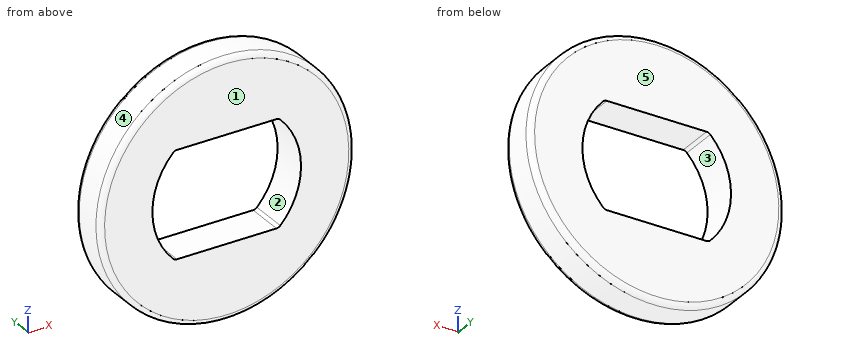
from build123d import *

# Parameters (mm, degrees)
SKETCH_1_R          = 12
EXTRUDE_1_DEPTH     = 3.5
CUT_EXTRUDE_1_DEPTH = 18.327723451
FILLET_1_R          = 0.5


with BuildPart() as part:
    # 草图1 → 凸台-拉伸1 (new body)
    with BuildSketch(Plane(origin=(0, 0, 0), x_dir=(1, 0, 0), z_dir=(0, 1, 0))):
        with Locations(Location((0, 0, 0), (0, 0, 270))):
            Circle(SKETCH_1_R)
    extrude(amount=EXTRUDE_1_DEPTH)

    # 草图2 → 切除-拉伸1 (cut, through all)
    with BuildSketch(Plane.XZ):
        with BuildLine():
            Line((4.898979486, -5), (-4.898979486, -5))
            ThreePointArc((-4.898979486, -5), (-7, 0), (-4.898979486, 5))
            Line((-4.898979486, 5), (4.898979486, 5))
            ThreePointArc((4.898979486, 5), (7, 0), (4.898979486, -5))
        make_face()
    extrude(amount=-CUT_EXTRUDE_1_DEPTH, mode=Mode.SUBTRACT)

    # 圆角1
    fillet_1_edges = [part.edges().sort_by_distance(p)[0] for p in [
        (4.898979486, 1.75, -5),
        (-4.898979486, 1.75, -5),
        (-4.898979486, 1.75, 5),
        (0, 0, -12),
        (0, 3.5, -12),
        (4.898979486, 1.75, 5),
    ]]
    fillet(fillet_1_edges, radius=FILLET_1_R)


solid = part.part
Can you work these out from the model? Positions are in its coordinate system, mm. Face numbers are marked on the shaded views. A direction names the side the tool comes from. Coordinates: 2 decimals unless noted, no trailing zeros. Write each loop counter-clockwise with the first axis right and the second up, starting at its lowest first coordinate (ties: lowest second). Pieces come first, ordered by that corner, then holes. Notation, with made-up numbers: (49.25, 45.5) -> (74.25, 45.5) arc R24 cw to (74.25, 77.5) -> close; hole circle Ø11 at (3.25, 23). An arc over 180 degrees is marked (long way). Write each question's results on one line, items separated by ' | '. Start each with the question number.
Q1. Imagine slicing it at A-A (y = 1). Write out the boundary of the cut face in (x, z), then the cut area to 3 significant figures.
Q2. Imagine slicing it at C-C (z = 0). Write out the boundary of the cut face in (x, y), then the cut area to 3 significant figures.
Q3. If I drill on probe 1 along X at (y, z) = (0.5, 0); probe 2 along X at (y, z) = (0.4, -2.25); probe 3 along Z at (x, y) = (4.25, 0.9), over which ranges is the centre line in solid material (lowest first)?
Q4. On a 3-axis mill with a long thin cutter (end or side, diameter ignored), from which of +Z, -Z, +X, -X, +Y, -Y can I reach the whole of each face in a straight line? I mean the marked faces 1 and 2. Say none if no direction works.
Q5. I'm going to push flat-ended pins straight in: pin 1 (2 mm diameter, centred on x = 8.5, y = 3, fed in from +Z); pin 2 (2 mm diameter, centred on y = 2.5, z = -9, fed in from +X). Where does each tip first touch, or does it pass through?
Q6. Imagine slicing it at B-B (x = 0). Write out the boundary of the cut face in (y, z).
Q7. We'd pull the mould along Z, two halves only. Please class the marked faces 3, 4 and 5: +Z half, -Z half, draft (parallel to the pull), parting line (faces both ways), or undercut.
Taken from the geometry:
1) outline: circle Ø24 at (0, 0); hole (-5.05, -4.85) arc R0.5 ccw to (-4.69, -5) -> (4.69, -5) arc R0.5 ccw to (5.05, -4.85) arc R7 ccw to (5.05, 4.85) arc R0.5 ccw to (4.69, 5) -> (-4.69, 5) arc R0.5 ccw to (-5.05, 4.85) arc R7 ccw to start | area: 325 mm^2
2) outline: (-12, 0.5) arc R0.5 ccw to (-11.5, 0) -> (-7, 0) -> (-7, 3.5) -> (-11.5, 3.5) arc R0.5 ccw to (-12, 3) -> close; (7, 0) -> (11.5, 0) arc R0.5 ccw to (12, 0.5) -> (12, 3) arc R0.5 ccw to (11.5, 3.5) -> (7, 3.5) -> close | area: 34.8 mm^2
3) probe 1: x = -12 to -7, 7 to 12 | probe 2: x = -11.78 to -6.63, 6.63 to 11.78 | probe 3: z = -11.22 to -5, 5 to 11.22
4) face 1: +Z, -Z, +X, -X, -Y | face 2: +Y, -Y
5) pin 1: stops at z = 9.37 | pin 2: stops at x = 8.94
6) outline: (0, -11.5) arc R0.5 ccw to (0.5, -12) -> (3, -12) arc R0.5 ccw to (3.5, -11.5) -> (3.5, -5) -> (0, -5) -> close; (0, 5) -> (3.5, 5) -> (3.5, 11.5) arc R0.5 ccw to (3, 12) -> (0.5, 12) arc R0.5 ccw to (0, 11.5) -> close
7) face 3: undercut | face 4: parting line | face 5: draft
